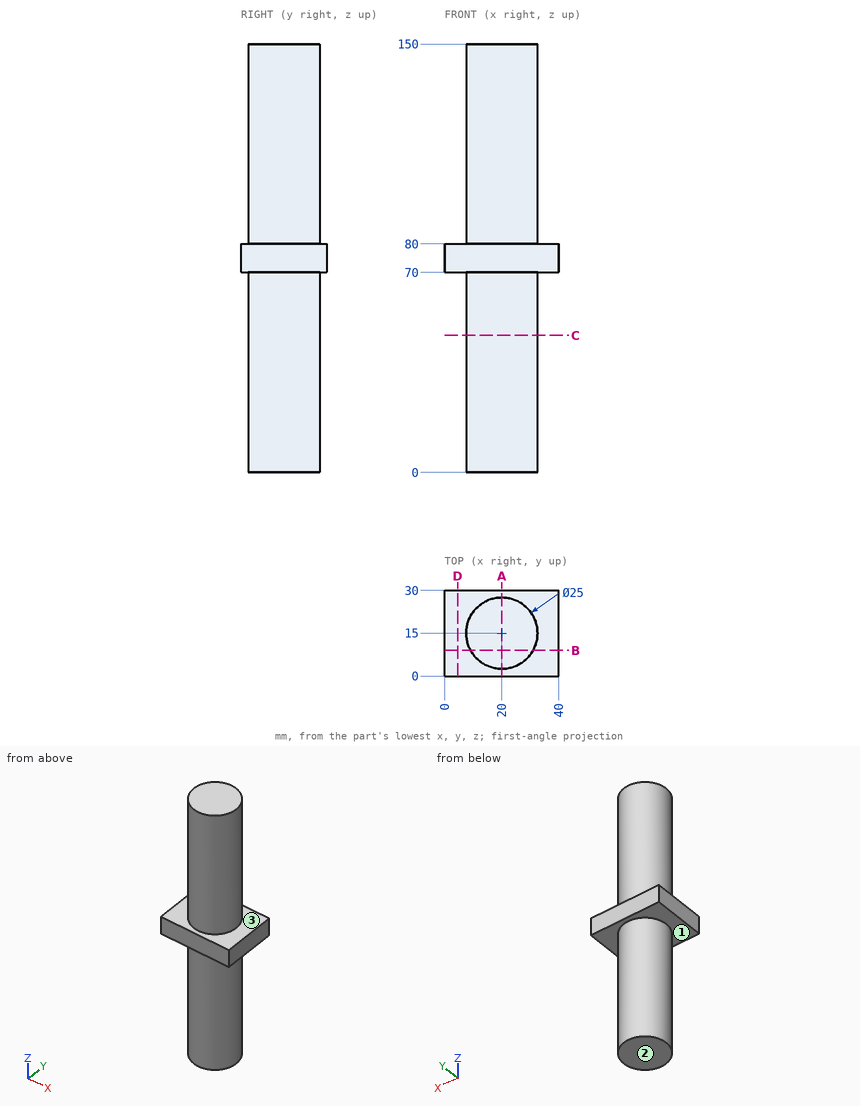
Input: dimensioned drawing with shaded views. Units: mm. Origin: part minimum x, y, z. A direction names the side the tool comes from. Coordinates: 2 decimals unless noted, no trailing zeros. Write each loop counter-clockwise with the first axis right and the second up, starting at its lowest first coordinate (ties: lowest second). Pieces come first, ordered by that corner, then holes. Notation, with made-up numbers: (14, 75) -> (41, 75) arc R28 ccw to (41, 106) -> close; hole circle Ø10 at (69.25, 52). An arc over 180 degrees is marked (long way). Return JSON: item names as keys, results as strings. Group by question number.
1) Set-up query: the marked faces 1, 2 and 3. Return all of +Z, -Z, +X, -X, +Y, -Y with unobstructed straight access to the full face (end or side cutting, diameter ignored); none if empty.
2) Section query B-B, the plane y = 9. Return loops of the section in (x, z).
3) Section query D-D, the plane x = 4.5. Return loops of the section in (y, z).
4) Contact query for flat-ended pins moving along their axis: P1, Ø6, axis at x = 26.5, y = 23.5, coming from the -Z side; P2, Ø2, axis at x = 23, z = 25, coming from the -Y side; P3, Ø4, axis at y = 5, z = 91.5, coming from the -X side; P4, Ø1.5, axis at x = 7.5, y = 6, coming from the -Z side. Output: stop coordinate, or through.
5) Section query A-A, the plane x = 20. Return loops of the section in (y, z), plus the area to 3 significant figures.
6) Section query C-C, the plane z = 48. Return loops of the section in (x, y).
7) Ray query, line 1 along Z through (x, y) = (33, 16.5); line 2 along X through (y, z) = (15, 61); line 3 along Y through (x, z) = (16, 102.5). Return the intervals inside material, ascending.
From the geometry:
{
 "1": {"face 1": "-Z", "face 2": "-Z, +X, -X, +Y, -Y", "face 3": "+Z"},
 "2": {"outline": "(0, 70) -> (9.03, 70) -> (9.03, 0) -> (30.97, 0) -> (30.97, 70) -> (40, 70) -> (40, 80) -> (30.97, 80) -> (30.97, 150) -> (9.03, 150) -> (9.03, 80) -> (0, 80) -> close"},
 "3": {"outline": "(0, 70) -> (30, 70) -> (30, 80) -> (0, 80) -> close"},
 "4": {"P1": "z = 0", "P2": "y = 2.66", "P3": "x = 10.4", "P4": "z = 70"},
 "5": {"outline": "(0, 70) -> (2.5, 70) -> (2.5, 0) -> (27.5, 0) -> (27.5, 70) -> (30, 70) -> (30, 80) -> (27.5, 80) -> (27.5, 150) -> (2.5, 150) -> (2.5, 80) -> (0, 80) -> close", "area": "3,800 mm²"},
 "6": {"outline": "circle Ø25 at (20, 15)"},
 "7": {"line 1": "70 to 80", "line 2": "7.5 to 32.5", "line 3": "3.16 to 26.84"}
}
